The figure shows three views and two pictorial views of one solid part (mm, origin at its lowest corner). Answer the questions. Give positions to 0.01 mm unless a question says otherwise; leave off trailing zeros. Loops run counter-clockwise (first coordinate to the right, second up) from the corner with the lowest first, then second, coordinate; pieces in that order, holes last. Notation, with made-up numbers: M 53,45.5 L 60,45.5 A33 ccw 60,73.5 Z; hole C -40,6.25 d9. An arc over 180 degrees is marked long. One line per item, written item: value. Start each with the question number.
Q1. A cutting plane is placed at C-C, the plane y = 22.5. Determine the outline of the cut face in (x, z).
Q2. A cutting plane is placed at D-D, the plane z = 2. Determine the outline of the cut face in (x, y).
Q3. Consider L1, parallel to X at y = 35.5, z = 19; L2, parallel to Y at x = 61.5, z = 20.5; L3, parallel to Z at x = 44, y = 10. Determine where each line is inside the solid, lowest interval first.
Q4. A flat-ended cylindrical pin translates along its axis: pin 1 (10 mm diameter, centred on x = 52, y = 27.5, fed in from +Z). Find the tip coordinate at first contact, or state that the pin passes through.
Q5. The mould has two halves that part along Y. Classify the marked faces 1, 2, 3 and 4: +Y half, -Y half, draft (parallel to the pull), parting line (faces both ways), or undercut.
Q6. A cutting plane is placed at A-A, the plane z = 22. Determine the outline of the cut face in (x, y).
Q7. A cutting plane is placed at B-B, the plane x = 52.5. Determine the outline of the cut face in (y, z).
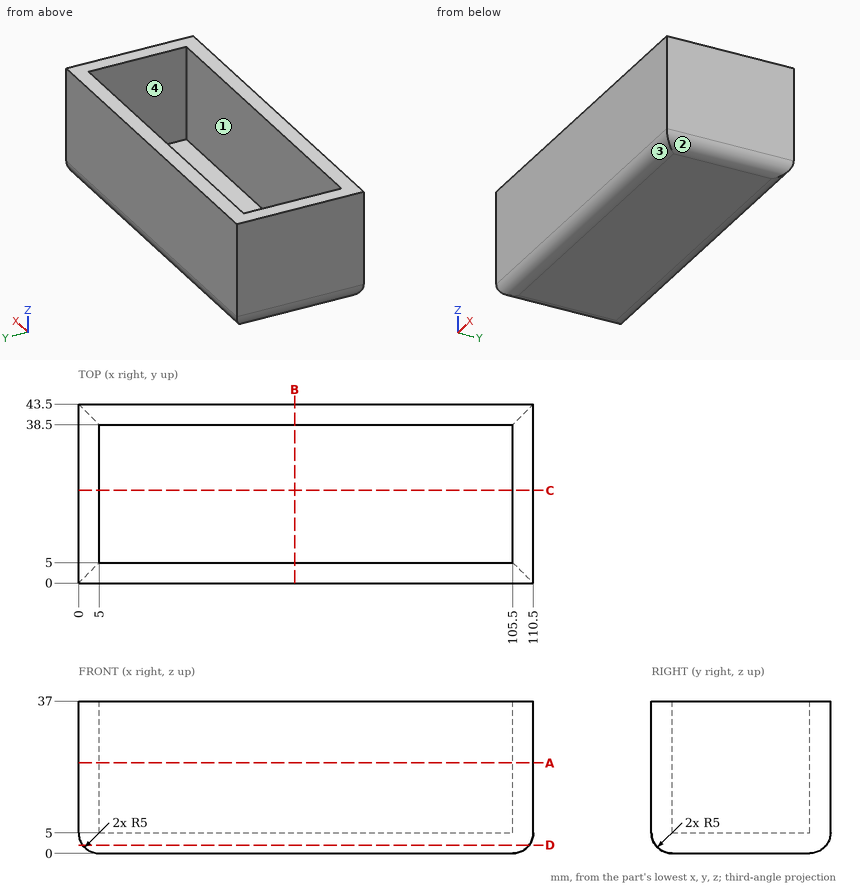
Answer block:
1. outline: M 0,5 A5 ccw 5,0 L 105.5,0 A5 ccw 110.5,5 L 110.5,37 L 105.5,37 L 105.5,5 L 5,5 L 5,37 L 0,37 Z
2. outline: M 1,1 L 109.5,1 L 109.5,42.5 L 1,42.5 Z
3. L1: 0 to 5, 105.5 to 110.5
3. L2: 0 to 5, 38.5 to 43.5
3. L3: 0 to 5
4. pin 1: z = 5
5. face 1: undercut
5. face 2: draft
5. face 3: -Y half
5. face 4: undercut
6. outline: M 0,0 L 110.5,0 L 110.5,43.5 L 0,43.5 Z; hole M 5,5 L 105.5,5 L 105.5,38.5 L 5,38.5 Z
7. outline: M 0,5 A5 ccw 5,0 L 38.5,0 A5 ccw 43.5,5 L 43.5,37 L 38.5,37 L 38.5,5 L 5,5 L 5,37 L 0,37 Z
